For this review, take the finished solid that the model builds, in its own axes (mm). A direction names the side the tool comes from. Coordinates: 2 decimals unless noted, no trailing zeros. Write each loop counter-clockwise with the first axis right and the second up, starting at its lowest first coordinate (ties: lowest second). Pieces come first, ordered by that corner, then holes.
```python
from build123d import *

# Parameters (mm, degrees)
SKETCH1_W           = 25.4
SKETCH1_H           = 25.4
SKETCH1_W_2         = 19.05
SKETCH1_H_2         = 19.05
BOSS_EXTRUDE1_DEPTH = 261.62
CUT_EXTRUDE2_DEPTH  = 264.156748726
SKETCH3_R           = 3.3734375
CUT_EXTRUDE3_DEPTH  = 264.156748726


with BuildPart() as part:
    # Sketch1 → Boss-Extrude1 (new body)
    with BuildSketch(Plane.XY):
        Rectangle(SKETCH1_W, SKETCH1_H)
        Rectangle(SKETCH1_W_2, SKETCH1_H_2, mode=Mode.SUBTRACT)
    extrude(amount=BOSS_EXTRUDE1_DEPTH)

    # Sketch2 → Cut-Extrude2 (cut, through all)
    with BuildSketch(Plane(origin=(12.7, 0, 0), x_dir=(0, 0, -1), z_dir=(1, 0, 0))):
        Polygon((-223.125170802, 12.7), (-261.62, -9.525), (-261.62, 12.7), align=None)
        Polygon((-38.494829198, 12.7), (0, -9.525), (0, 12.7), align=None)
    extrude(amount=-CUT_EXTRUDE2_DEPTH, mode=Mode.SUBTRACT)

    # Sketch3 → Cut-Extrude3 (cut, through all)
    with BuildSketch(Plane.XZ.offset(12.7)):
        with Locations(Location((0, 252.095, 0), (0, 0, 270))):
            Circle(SKETCH3_R)
        with Locations(Location((0, 236.22, 0), (0, 0, 270))):
            Circle(SKETCH3_R)
        with Locations(Location((0, 25.4, 0), (0, 0, 270))):
            Circle(SKETCH3_R)
        with Locations(Location((0, 9.525, 0), (0, 0, 270))):
            Circle(SKETCH3_R)
    extrude(amount=-CUT_EXTRUDE3_DEPTH, mode=Mode.SUBTRACT)


solid = part.part
```
Q1. Add section D-D (y = -6.75). State the section outline as (x, z) points (3 decimals).
Ans:
outline: (-12.7, 4.806) - (-9.525, 4.806) - (-9.525, 256.814) - (-12.7, 256.814) - close; (9.525, 4.806) - (12.7, 4.806) - (12.7, 256.814) - (9.525, 256.814) - close
Q2. Add section C-C (z = 25.4). State the section outline as (x, y) points (3 decimals), then the cut area to 3 significant figures.
Ans:
outline: (-12.7, -12.7) - (-3.373, -12.7) - (-3.373, -9.525) - (-9.525, -9.525) - (-9.525, 5.14) - (-12.7, 5.14) - close; (3.373, -12.7) - (12.7, -12.7) - (12.7, 5.14) - (9.525, 5.14) - (9.525, -9.525) - (3.373, -9.525) - close
area: 152 mm2
Q3. Tool access review of faces 4 (the flat face through (-9.525, 0, 129)), 5 (the flat face through (0, -12.7, 129)): name each direction out of +Z, -Z, +X, -X, +Y, -Y from which nothing blocks a thin tool from reaching the whole face with its end or side.
Ans:
face 4: +Z, -Z
face 5: +Z, -Z, +X, -X, -Y
Q4. Draft analysis for pull direction X (two halves, no side actions). For faces 1 (the flat face through (-0.88, 9.87, 228.03)), 2 (the flat face through (0, -9.525, 129)), 3 (the flat face through (-12.7, 0, 129)), state which applies: +X half, -X half, draft (parallel to the pull), parting line (faces both ways), or undercut.
Ans:
face 1: draft
face 2: undercut
face 3: -X half
Q5. Clearance check with a flat-ended pin moving along its axis: pin 1 Ø6 at (x, y) = (9, 5.5) entering from -Z. State where the tip first meets the part, or that it passes through.
Ans:
pin 1: stops at z = 20.91
Q6. Add section A-A (z = 106). State the section outline as (x, y) points (3 decimals).
Ans:
outline: (-12.7, -12.7) - (12.7, -12.7) - (12.7, 12.7) - (-12.7, 12.7) - close; hole (-9.525, -9.525) - (9.525, -9.525) - (9.525, 9.525) - (-9.525, 9.525) - close
Q7. For probe 1 along Y at (x, z) = (0.25, 106.5) (3 decimals); probe 2 along X at (y, z) = (-11.3, 236.22), list the stretches that pass through material, from the lowest coordinate up.
Ans:
probe 1: y = -12.7 to -9.525, 9.525 to 12.7
probe 2: x = -12.7 to -3.37, 3.37 to 12.7
Q8. Add section B-B (y = 3.75). State the section outline as (x, z) points (3 decimals), then the cut area to 3 significant figures.
Ans:
outline: (-12.7, 22.993) - (-9.525, 22.993) - (-9.525, 238.627) - (-12.7, 238.627) - close; (9.525, 22.993) - (12.7, 22.993) - (12.7, 238.627) - (9.525, 238.627) - close
area: 1,370 mm2
